```python
from build123d import *

# Parameters (mm, degrees)
F1_DEPTH = 200
F3_DEPTH = 150
F4_W     = 40
F4_H     = 120
F4_W_2   = 30
F5_DEPTH = 150
F6_R     = 19.99999
F7_R     = 15
F7_R_2   = 14.99999


# Not quite as in the source:
# - a fillet or chamfer is up to 0.001 mm smaller than in the source, because OpenCascade refuses the exact size
# - ends of sketch curves that miss each other by under 0.0002 mm in the source are joined


with BuildPart() as f1:
    # F0 (on Top) → F1 (new body)
    with BuildSketch(Plane.XY):
        with BuildLine():
            Line((-203.32088, 103.750296), (-260.740998, 72.83177))
            ThreePointArc((-260.740998, 72.83177), (-264.5851610502, 69.1549250028), (-266, 64.027059))
            Line((-266, 64.027059), (-266, -64.027059))
            ThreePointArc((-266, -64.027059), (-264.5851610502, -69.1549250028), (-260.7409980515, -72.8317700956))
            Line((-260.7409980515, -72.8317700956), (-203.32088, -103.750296))
            ThreePointArc((-203.32088, -103.750296), (-103.8608632236, -129.7071209998), (-1.082674041, -131.348924606))
            Line((-1.082674041, -131.348924606), (214.09118, -102.064591))
            ThreePointArc((214.09118, -102.064591), (251.1966304028, -82.0748460353), (266, -42.612654))
            Line((266, -42.612654), (266, 42.612654))
            ThreePointArc((266, 42.612654), (251.1966304028, 82.0748460353), (214.0911799923, 102.0645909435))
            Line((214.0911799923, 102.0645909435), (-1.082674, 131.348925))
            ThreePointArc((-1.082674, 131.348925), (-103.8608632236, 129.7071209998), (-203.32088, 103.750296))
        make_face()
    extrude(amount=F1_DEPTH)

    # F2 (on Front) → F3 (cut, symmetric)
    with BuildSketch(Plane.XZ):
        Polygon((266, 200), (-266, 200), (-266, 153), align=None)
    extrude(amount=F3_DEPTH, both=True, mode=Mode.SUBTRACT)

    # F4 (on Front) → F5 (cut, symmetric)
    with BuildSketch(Plane.XZ):
        with Locations((126, 60)):
            Rectangle(F4_W, F4_H)
        with Locations((-89, 60)):
            Rectangle(F4_W_2, F4_H)
    extrude(amount=F5_DEPTH, both=True, mode=Mode.SUBTRACT)

    # F6 (radius 20 in the source; OpenCascade refuses exactly that, so slightly less here)
    f6_edges = [f1.edges().sort_by_distance(p)[0] for p in [
        (146, 0, 120),
        (106, 0, 120),
    ]]
    fillet(f6_edges, radius=F6_R)

    # F7 (call 1 of 2: OpenCascade refuses the feature's edges together)
    f7_edges = [f1.edges().sort_by_distance(p)[0] for p in [
        (-74, 0, 120),
    ]]
    fillet(f7_edges, radius=F7_R)

    # F7#2 (call 2 of 2) (radius 15 in the source; OpenCascade refuses exactly that, so slightly less here)
    f7_2_edges = [f1.edges().sort_by_distance(p)[0] for p in [
        (-104, 0, 120),
    ]]
    fillet(f7_2_edges, radius=F7_R_2)


solid = f1.part
```
For this review, take the finished solid that the model builds, in its own axes (mm). A direction names the side the tool comes from. Coordinates: 2 decimals unless noted, no trailing zeros. Loops run counter-clockwise (first coordinate to the right, second up) from the corner with the lowest first, then second, coordinate; pieces in that order, holes last. Notation, with made-up numbers: (23, -26) -> (73, -26) arc R10 ccw to (73, -12) -> close; hole circle Ø4 at (59, -28). An arc over 180 degrees is marked (long way). Return JSON: item names as keys, results as strings. Group by question number.
(1) Consider section C-C, the plane z = 139.5. Give the boundary of the cut face in (x, y), plus the area to 3 significant figures.
(2) Tool access review of faces 1 (the flat face through (146, 2, 49)), 2 (the flat face through (15, 2, 0)): name each direction out of +Z, -Z, +X, -X, +Y, -Y from which nothing blocks a thin tool from reaching the whole face with its end or side.
(3) Mouldability with a two-part tool opening along X and no side actions: class faces 3 (the cylindrical face through (251.59, 81.62, 98.6)), 4 (the cylindrical face through (-125.037, 126.278, 86.967)), 5 (the flat face through (106, 2, 49)) as pulls with the +X half, pulls with the -X half, needs draft (parallel to the pull), parting line crosses it, or undercut.
(4) Consider section D-D, the plane x = 65. Give the boundary of the cut face in (y, z).
(5) For pin 1 Ø10 at (x, y) = (-204.5, 56) entering from -Z; pin 2 Ø1 at (x, z) = (-95.5, 140) entering from +Y; pin 3 Ø10 at (y, z) = (55.5, 46) entering from +X; pin 4 Ø4 at (x, z) = (178, 43.5) entering from +Y, all flat-tipped, find the tip position at first contact; note any pin that passes through.
(6) To check wall thickness, follow L1, parallel to X at y = -82, z = 61; L2, parallel to X at y = -76, z = 100.5; L3, parallel to Y at x = -19.5, z = 165. State the ranges of each line that lie inside material, in increasing order.
(7) Consider section A-A, the plane z = 61. Give the boundary of the cut face in (x, y), plus the area to 3 significant figures.
Results below:
{
 "1": {"outline": "(-266, -64.03) arc R10 ccw to (-260.74, -72.83) -> (-203.32, -103.75) arc R430.56 ccw to (-1.08, -131.35) -> (214.09, -102.06) arc R60 ccw to (266, -42.61) -> (266, 42.61) arc R60 ccw to (214.09, 102.06) -> (-1.08, 131.35) arc R430.56 ccw to (-203.32, 103.75) -> (-260.74, 72.83) arc R10 ccw to (-266, 64.03) -> close", "area": "121,000 mm2"},
 "2": {"face 1": "-Z, +Y, -Y", "face 2": "-Z, +X, -X, +Y, -Y"},
 "3": {"face 3": "pulls with the +X half", "face 4": "parting line crosses it", "face 5": "undercut"},
 "4": {"outline": "(-122.36, 0) -> (122.36, 0) -> (122.36, 182.24) -> (-122.36, 182.24) -> close"},
 "5": {"pin 1": "stops at z = 0", "pin 2": "stops at y = 130.82", "pin 3": "stops at x = 265.48", "pin 4": "stops at y = 107.25"},
 "6": {"L1": "x = -243.71 to -104, -74 to 106, 146 to 251.26", "L2": "x = -254.86 to -104, -74 to 106.01, 145.99 to 255.85", "L3": "y = -132.87 to 132.87"},
 "7": {"outline": "(-266, -64.03) arc R10 ccw to (-260.74, -72.83) -> (-203.32, -103.75) arc R430.56 ccw to (-104, -129.69) -> (-104, 129.69) arc R430.56 ccw to (-203.32, 103.75) -> (-260.74, 72.83) arc R10 ccw to (-266, 64.03) -> close; (-74, -132.73) arc R430.56 ccw to (-1.08, -131.35) -> (106, -116.78) -> (106, 116.78) -> (-1.08, 131.35) arc R430.56 ccw to (-74, 132.73) -> close; (146, -111.33) -> (214.09, -102.06) arc R60 ccw to (266, -42.61) -> (266, 42.61) arc R60 ccw to (214.09, 102.06) -> (146, 111.33) -> close", "area": "104,000 mm2"}
}
